Here's the drawing with two shaded views (mm, measured from the low corner). I have some questions. Coordinates: 2 decimals unless noted, no trailing zeros. Loops run counter-clockwise (first coordinate to the right, second up) from the corner with the lowest first, then second, coordinate; pieces in that order, holes last. Notation, with made-up numbers: (2.25, 31.5) -> (16.25, 31.5) arc R7 ccw to (16.25, 36.5) -> close; hole circle Ø6 at (-12.75, 37). An arc over 180 degrees is marked (long way). Answer as a JSON object with one key per item and string values. Group by question number.
Q1. I need wall thicknesses on line 1 (Z direction, x = 76, y = 44); line 2 (Z direction, x = 15, y = 48); line 3 (Y direction, x = 34, z = 24.5). Which ranges of each line are inside material? Lowest first, please.
Q2. I want a section at D-D on y = 51. Write out the boundary of the cut face in (x, z), then the cut area to 3 significant figures.
Q3. I want a section at A-A on y = 38.5. Write out the boundary of the cut face in (x, z), then the cut area to 3 significant figures.
Q4. I want a section at C-C on x = 21. Write out the boundary of the cut face in (y, z), then the cut area to 3 significant figures.
Q5. I'm going to push flat-ended pins straight in: pin 1 (5 mm diameter, centred on x = 13, z = 45, fed in from -Y); pin 2 (8 mm diameter, centred on y = 34, z = 44, fed in from -X); pin 3 (1 mm diameter, centred on x = 20, y = 24.5, fed in from +Z); pin 4 (5 mm diameter, centred on x = 16.5, y = 15.5, fed in from -Z). Where does each tip first touch, or does it pass through?
Q6. I want a section at B-B on z = 33.5. Write out the boundary of the cut face in (x, y), then the cut area to 3 significant figures.
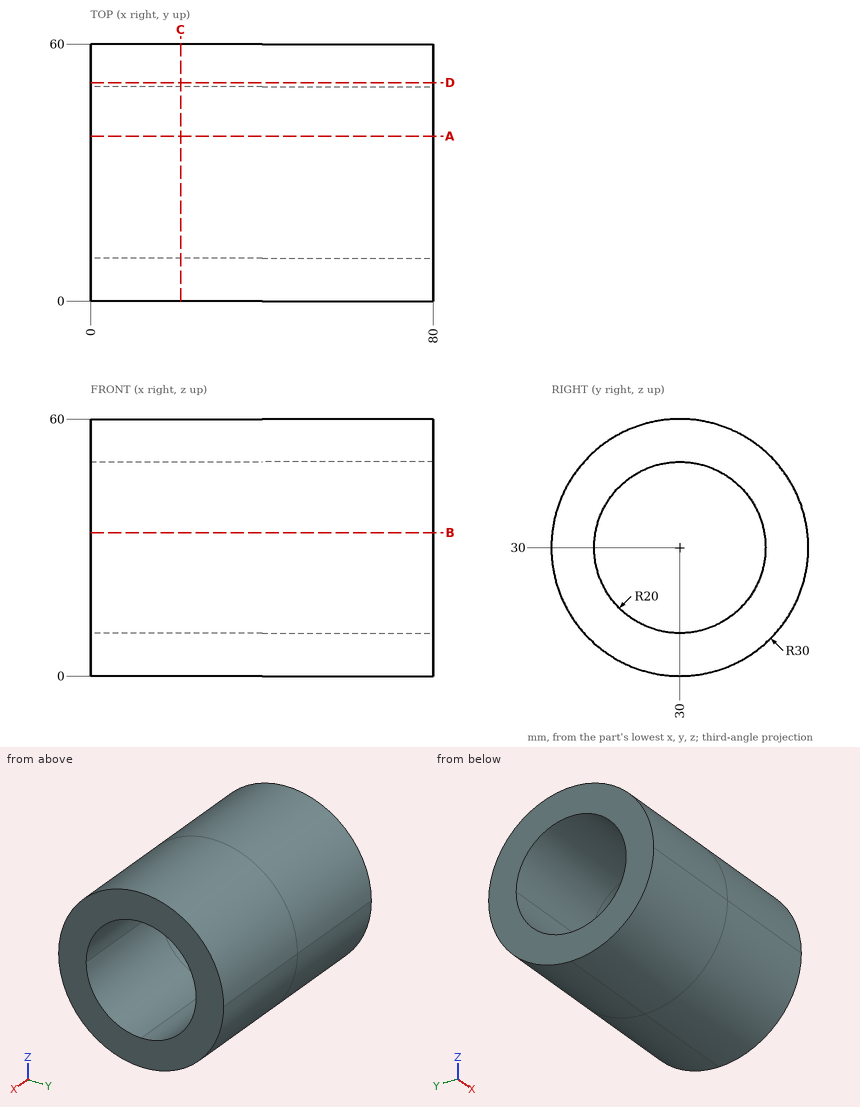
Result set:
{
 "1": {"line 1": "z = 3.47 to 15.72, 44.28 to 56.53", "line 2": "z = 6 to 21.28, 38.72 to 54", "line 3": "y = 0.51 to 10.77, 49.23 to 59.49"},
 "2": {"outline": "(0, 8.58) -> (80, 8.58) -> (80, 51.42) -> (0, 51.42) -> close", "area": "3,430 mm²"},
 "3": {"outline": "(0, 1.23) -> (80, 1.23) -> (80, 11.9) -> (0, 11.9) -> close; (0, 48.1) -> (80, 48.1) -> (80, 58.77) -> (0, 58.77) -> close", "area": "1,710 mm²"},
 "4": {"outline": "circle Ø60 at (30, 30); hole circle Ø40 at (30, 30)", "area": "1,570 mm²"},
 "5": {"pin 1": "stops at y = 2.73", "pin 2": "passes through", "pin 3": "stops at z = 59.58", "pin 4": "stops at z = 2.5"},
 "6": {"outline": "(0, 0.2) -> (80, 0.2) -> (80, 10.31) -> (0, 10.31) -> close; (0, 49.69) -> (80, 49.69) -> (80, 59.8) -> (0, 59.8) -> close", "area": "1,620 mm²"}
}
